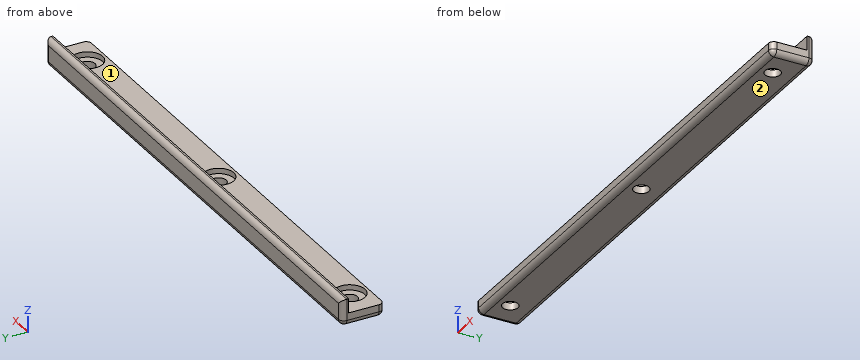
```python
from build123d import *

# Parameters (mm, degrees)
SKETCH1_W                = 150
SKETCH1_H                = 10
SKETCH1_R                = 4.25
BOSS_EXTRUDE1_DEPTH      = 1.5
SKETCH2_W                = 150
SKETCH2_H                = 10
SKETCH2_R                = 2.15
BOSS_EXTRUDE2_DEPTH      = 2
BOSS_EXTRUDE3_DEPTH      = 4
BOSS_EXTRUDE3_DEPTH_BACK = 3.5
SKETCH3_W                = 150
SKETCH3_H                = 2
FILLET1_R                = 1.5


with BuildPart() as part:
    # Sketch1 → Boss-Extrude1 (new body)
    with BuildSketch(Plane.XY):
        with Locations((75, -5)):
            Rectangle(SKETCH1_W, SKETCH1_H)
        with Locations((75, -5)):
            Circle(SKETCH1_R, mode=Mode.SUBTRACT)
        with Locations((141.5, -5)):
            Circle(SKETCH1_R, mode=Mode.SUBTRACT)
        with Locations((8.5, -5)):
            Circle(SKETCH1_R, mode=Mode.SUBTRACT)
    extrude(amount=BOSS_EXTRUDE1_DEPTH)

    # Sketch2 → Boss-Extrude2 (add)
    with BuildSketch(Plane(origin=(0, 0, 0), x_dir=(-1, 0, 0), z_dir=(0, 0, -1))):
        with Locations((-75, -5)):
            Rectangle(SKETCH2_W, SKETCH2_H)
        with Locations((-8.5, -5)):
            Circle(SKETCH2_R, mode=Mode.SUBTRACT)
        with Locations((-75, -5)):
            Circle(SKETCH2_R, mode=Mode.SUBTRACT)
        with Locations((-141.5, -5)):
            Circle(SKETCH2_R, mode=Mode.SUBTRACT)
    extrude(amount=BOSS_EXTRUDE2_DEPTH)

    # Sketch3 → Boss-Extrude3 (add, two sides: drawn at the far end of the back side and taken through both)
    with BuildSketch(Plane.XY.offset(1.5).offset(-BOSS_EXTRUDE3_DEPTH_BACK)):
        with Locations((75, 1)):
            Rectangle(SKETCH3_W, SKETCH3_H)
    extrude(amount=BOSS_EXTRUDE3_DEPTH + BOSS_EXTRUDE3_DEPTH_BACK)

    # Fillet1
    fillet1_edges = [part.edges().sort_by_distance(p)[0] for p in [
        (150, -4, -2),
        (75, -10, -2),
        (0, -4, -2),
        (0, 2, 1.75),
        (75, 2, -2),
        (150, 2, 1.75),
        (75, 2, 5.5),
        (150, -10, -0.25),
        (0, -10, -0.25),
    ]]
    fillet(fillet1_edges, radius=FILLET1_R)


solid = part.part
```
Source: CAD feature listing. Evaluate the final solid. Frame: model axes, mm. Face numbers are marked on the shaded views. A direction names the side the tool comes from. Coordinates: 2 decimals unless noted, no trailing zeros. Write each loop counter-clockwise with the first axis right and the second up, starting at its lowest first coordinate (ties: lowest second). Pieces come first, ordered by that corner, then holes. Notation, with made-up numbers: M 14.25,29 L 73.25,29 A19 ccw 73.25,48 Z; hole C 77,76.5 d5. An arc over 180 degrees is marked long. Answer as a JSON object with one key per item and string values.
1. Ray query, L1, parallel to Y at x = 8.5, z = 0.65; L2, parallel to Y at x = 8.5, z = -0.5; L3, parallel to Z at x = 12, y = -3.5. Return the intervals inside material, ascending.
Evaluation:
{"L1": "-10 to -9.25, -0.75 to 2", "L2": "-10 to -7.15, -2.85 to 2", "L3": "-2 to 0"}
2. Cut plane B-B on y = -5. State how many separate pieces and enclosed holes the cut face has, plus the area to 3 significant figures.
Evaluation:
{"separate pieces": "4", "enclosed holes": "0", "area": "460 mm^2"}
3. Contact query for flat-ended pins moving along their axis: P1, Ø4, axis at x = 8.5, y = -5, coming from the -Z side; P2, Ø4, axis at x = 40.5, y = -8, coming from the +Z side; P3, Ø3, axis at x = 106.5, z = 3.5, coming from the -Y side; P4, Ø5.5, axis at x = 141.5, y = -5, coming from the +Z side. Output: stop coordinate, or through.
Evaluation:
{"P1": "through", "P2": "z = 1.5", "P3": "y = 0", "P4": "z = 0"}
4. Cut plane A-A on x = 8.5. Output: boundary loops of the cut face in (y, z).
Evaluation:
{"outline": "M -10,-0.5 A1.5 ccw -8.5,-2 L -7.15,-2 L -7.15,0 L -9.25,0 L -9.25,1.5 L -10,1.5 Z; M -2.85,-2 L 0.5,-2 A1.5 ccw 2,-0.5 L 2,4 A1.5 ccw 0.5,5.5 L 0,5.5 L 0,1.5 L -0.75,1.5 L -0.75,0 L -2.85,0 Z"}
5. Cut plane C-C on x = 62. Output: boundary loops of the cut face in (y, z), plus the area to 3 significant figures.
Evaluation:
{"outline": "M -10,-0.5 A1.5 ccw -8.5,-2 L 0.5,-2 A1.5 ccw 2,-0.5 L 2,4 A1.5 ccw 0.5,5.5 L 0,5.5 L 0,1.5 L -10,1.5 Z", "area": "48.6 mm^2"}
6. Access query for the marked faces 1 and 2. Directions: +Z, -Z, +X, -X, +Y, -Y. A direction counts if a zero-diameter tool reaches every point of the face in a straight line with its end or side. Return the directions, or none.
Evaluation:
{"face 1": "+Z, +X, -X, -Y", "face 2": "-Z, +X, -X, +Y, -Y"}
